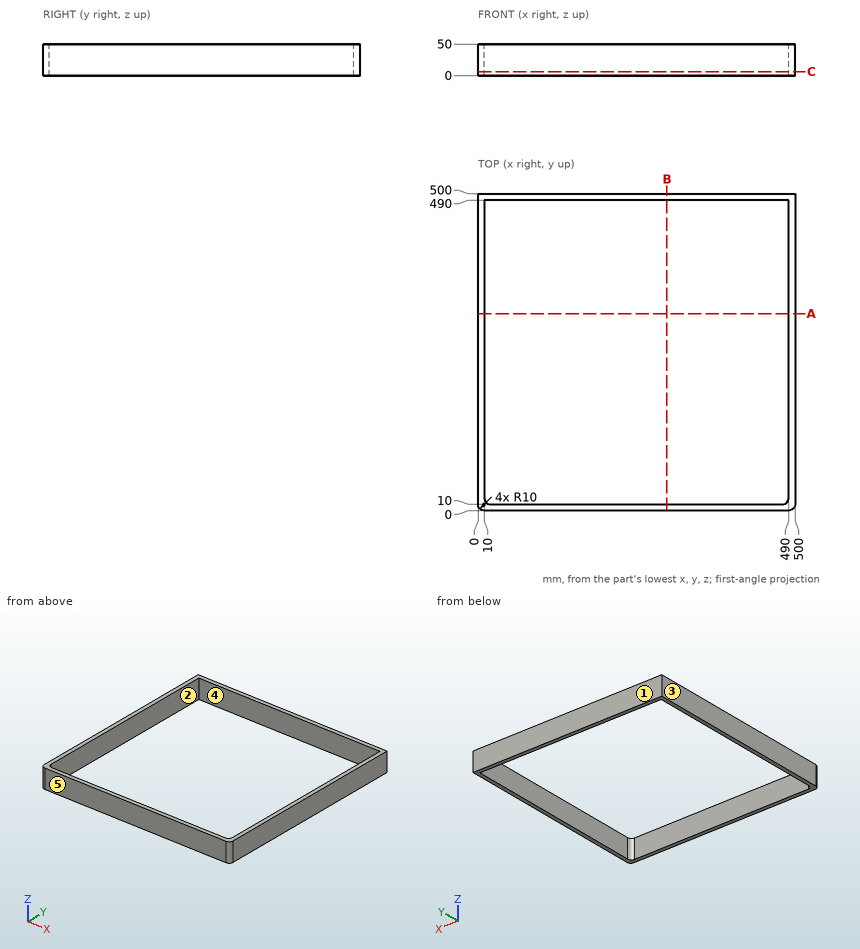
The figure shows three views and two pictorial views of one solid part (mm, origin at its lowest corner). Answer the questions. A direction names the side the tool comes from. Coordinates: 2 decimals unless noted, no trailing zeros. Loops run counter-clockwise (first coordinate to the right, second up) from the corner with the lowest first, then second, coordinate; pieces in that order, holes last.
(1) The part is cut by section A-A (y = 311). Determine the outline of the cut face in (x, z).
Solution:
outline: (0, 0) - (10, 0) - (10, 50) - (0, 50) - close; (490, 0) - (500, 0) - (500, 50) - (490, 50) - close
(2) The part is cut by section C-C (z = 6.5). Determine the outline of the cut face in (x, y).
Solution:
outline: (0, 10) arc R10 ccw to (10, 0) - (490, 0) arc R10 ccw to (500, 10) - (500, 500) - (0, 500) - close; hole (10, 20) arc R10 ccw to (20, 10) - (480, 10) arc R10 ccw to (490, 20) - (490, 490) - (10, 490) - close
(3) A tool of negligible diameter and unlimited length cuts with its end or side. For the marked faces 1 and 2, from which of +Z, -Z, +X, -X, +Y, -Y can it reach the whole face along a straight path? Write none if from no direction.
Solution:
face 1: +Z, -Z, +X, -X, +Y
face 2: +Z, -Z
(4) The mould has two halves that part along X. Classify the marked faces 3, 4 and 5: released by +X, released by -X, zero draft, split by the parting line, or undercut.
Solution:
face 3: released by -X
face 4: undercut
face 5: zero draft
(5) Consider line 1 along Y through (x, z) = (213, 46.5). Determine where the line is inside the solid, lowest interval first.
Solution:
line 1: y = 0 to 10, 490 to 500
